Geometry: final body of the model. Coordinates: model frame, mm. Face numbers are marked on the shaded views. A direction names the side the tool comes from. Give positions to 0.01 mm unless a question says otherwise; leave off trailing zeros. Write each loop counter-clockwise with the first axis right and the second up, starting at its lowest first coordinate (ties: lowest second). Pieces come first, ordered by that corner, then holes. Notation, with made-up numbers: (61, 51.5) -> (69, 51.5) arc R22 ccw to (69, 76.5) -> close; hole circle Ø9 at (-36, 25.5). An arc over 180 degrees is marked (long way). Answer as a JSON object with one key per item and string values.
from build123d import *

# Parameters (mm, degrees)
ESQUISSE1_W        = 196.2
ESQUISSE1_H        = 72.3
ESQUISSE1_W_2      = 192.2
ESQUISSE1_H_2      = 68.3
BOSS_EXTRU_1_DEPTH = 28.8
ESQUISSE1_3_W      = 192.2
ESQUISSE1_3_H      = 68.3
ESQUISSE1_3_R      = 2
BOSS_EXTRU_2_DEPTH = 2


with BuildPart() as part:
    # Esquisse1 → Boss.-Extru.1 (new body)
    with BuildSketch(Plane(origin=(0, 0, 0), x_dir=(1, 0, 0), z_dir=(0, 1, 0))):
        with Locations((98.1, 36.15)):
            Rectangle(ESQUISSE1_W, ESQUISSE1_H)
        with Locations((98.1, 36.15)):
            Rectangle(ESQUISSE1_W_2, ESQUISSE1_H_2, mode=Mode.SUBTRACT)
    extrude(amount=BOSS_EXTRU_1_DEPTH)

    # Esquisse1<3> → Boss.-Extru.2 (add)
    with BuildSketch(Plane(origin=(0, 0, 0), x_dir=(1, 0, 0), z_dir=(0, 1, 0))):
        with Locations((98.1, 36.15)):
            Rectangle(ESQUISSE1_3_W, ESQUISSE1_3_H)
        with Locations(Location((29.6, 55.65, 0), (0, 0, 270))):
            Circle(ESQUISSE1_3_R, mode=Mode.SUBTRACT)
        with Locations(Location((29.6, 16.65, 0), (0, 0, 90))):
            Circle(ESQUISSE1_3_R, mode=Mode.SUBTRACT)
        with Locations(Location((166.6, 55.65, 0), (0, 0, 90))):
            Circle(ESQUISSE1_3_R, mode=Mode.SUBTRACT)
        with Locations(Location((166.6, 16.65, 0), (0, 0, 270))):
            Circle(ESQUISSE1_3_R, mode=Mode.SUBTRACT)
    extrude(amount=BOSS_EXTRU_2_DEPTH)


solid = part.part
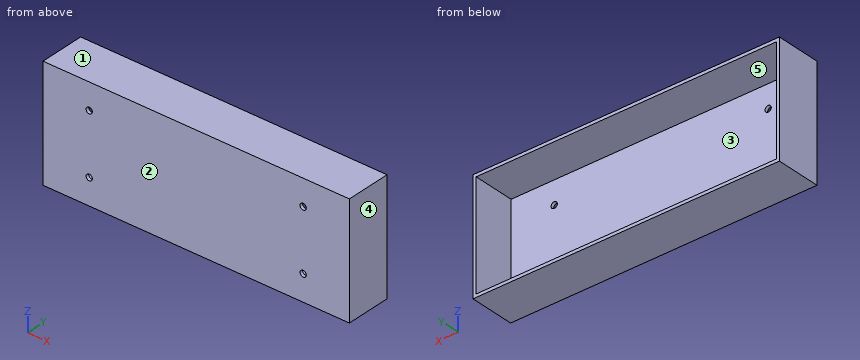
Q1. Cut plane B-B (y = 23). Return the cut outline in (x, z).
Values:
{"outline": "(0, -72.3) -> (196.2, -72.3) -> (196.2, 0) -> (0, 0) -> close; hole (2, -70.3) -> (194.2, -70.3) -> (194.2, -2) -> (2, -2) -> close"}
Q2. Cut plane A-A (z = -16.65). Return the cut outline in (x, y).
Values:
{"outline": "(0, 0) -> (27.6, 0) -> (27.6, 2) -> (2, 2) -> (2, 28.8) -> (0, 28.8) -> close; (31.6, 0) -> (164.6, 0) -> (164.6, 2) -> (31.6, 2) -> close; (168.6, 0) -> (196.2, 0) -> (196.2, 28.8) -> (194.2, 28.8) -> (194.2, 2) -> (168.6, 2) -> close"}
Q3. Mould query, pull axis Z, two halves, no side actions, for the marked faces 1, 2 and 3. Classes: pulls with the +Z half, pulls with the -Z half, needs draft (parallel to the pull), parting line crosses it, or undercut.
Values:
{"face 1": "pulls with the +Z half", "face 2": "needs draft", "face 3": "undercut"}
Q4. Material intervals for L1, parallel to X at y = 1.1, z = -16.65; L2, parallel to Z at x = 166.6, y = 1.55; L3, parallel to Z at x = 122, y = 19.25, sorted ascending. Write a range as from..to.
Values:
{"L1": "0..27.6, 31.6..164.6, 168.6..196.2", "L2": "-72.3..-57.65, -53.65..-18.65, -14.65..0", "L3": "-72.3..-70.3, -2..0"}
Q5. Cut plane D-D (x = 92.5). Return the cut outline in (y, z).
Values:
{"outline": "(0, -72.3) -> (28.8, -72.3) -> (28.8, -70.3) -> (2, -70.3) -> (2, -2) -> (28.8, -2) -> (28.8, 0) -> (0, 0) -> close"}
Q6. Cut plane C-C (x = 166.6). Return the cut outline in (y, z), and give its area (3 significant figures).
Values:
{"outline": "(0, -72.3) -> (28.8, -72.3) -> (28.8, -70.3) -> (2, -70.3) -> (2, -57.65) -> (0, -57.65) -> close; (0, -53.65) -> (2, -53.65) -> (2, -18.65) -> (0, -18.65) -> close; (0, -14.65) -> (2, -14.65) -> (2, -2) -> (28.8, -2) -> (28.8, 0) -> (0, 0) -> close", "area": "236 mm²"}
Q7. Set-up query: the marked faces 4 and 5. Return all of +Z, -Z, +X, -X, +Y, -Y with unobstructed straight access to the full face (end or side cutting, diameter ignored); none if empty.
Values:
{"face 4": "+Z, -Z, +X, +Y, -Y", "face 5": "+Y"}
Q8. First-contact query: P1, Ø5, axis at y = 25, z = -25, coming from the -X side; P2, Ø4, axis at x = 105.5, z = -42, coming from the +Y side. Flat tips, straight axial feed; report the tip coordinate or a pass-through.
Values:
{"P1": "x = 0", "P2": "y = 2"}
